from build123d import *

# Parameters (mm, degrees)
F1_DEPTH = 12.7
F4_SIZE  = 0.5
F6_R     = 7.25
F7_DEPTH = 9.3323626992
F8_SIZE  = 0.5


# Not quite as in the source:
# - a feature names something its author has since deleted; it is built from what else it names


with BuildPart() as f1:
    # F0 (on Right) → F1 (new body, symmetric)
    with BuildSketch(Plane.YZ):
        Polygon((12.7, 76.2), (-12.7, 76.2), (-12.7, 60.325), (-3.302, 60.325), (-3.302, 69.85), (0, 69.85), (0, -76.2), (12.7, -76.2), align=None)
    extrude(amount=F1_DEPTH, both=True)

    # F2 (on Right) → F3 (revolve)
    with BuildSketch(Plane.YZ):
        Polygon((-77.6932350437, -23.067179641), (-79.3034106209, -26.5202123096), (6.35, -66.4610536293), (7.9601755772, -63.0080209607), align=None)
    revolve(axis=Axis((0, -36.4767053105, -46.4906329695), (0, 0.906307787, -0.4226182617)))

    # F4
    f4_edges = [f1.edges().sort_by_distance(p)[0] for p in [
        (-12.7, 0, 76.2),
        (-12.7, 0, -3.175),
        (-12.7, 6.35, -76.2),
        (-12.7, -1.651, 69.85),
        (-12.7, -3.302, 65.0875),
        (-12.7, -12.7, 68.2625),
        (-12.7, -8.001, 60.325),
        (12.7, 6.35, -76.2),
        (12.7, 0, 76.2),
        (12.7, -12.7, 68.2625),
        (12.7, -1.651, 69.85),
        (12.7, -3.302, 65.0875),
        (12.7, -8.001, 60.325),
        (12.7, 0, -3.175),
        (0, 0, -76.2),
        (0, -12.7, 76.2),
        (0, -12.7, 60.325),
        (0, -3.302, 60.325),
    ]]
    chamfer(f4_edges, length=F4_SIZE)

    # F6 (on offset) → F7 (join, up to face)
    with BuildSketch(Plane(origin=(0, 19.834208268, -9.2488432088), x_dir=(1, 0, 0), z_dir=(0, -0.906307787, 0.4226182617))):
        with Locations((0, -57.5505444768)):
            Circle(F6_R)
    extrude(amount=-F7_DEPTH)

    # F8
    f8_edges = [f1.edges().sort_by_distance(p)[0] for p in [
        (-7.25, -4.487703, -61.40735),
    ]]
    chamfer(f8_edges, length=F8_SIZE)


solid = f1.part
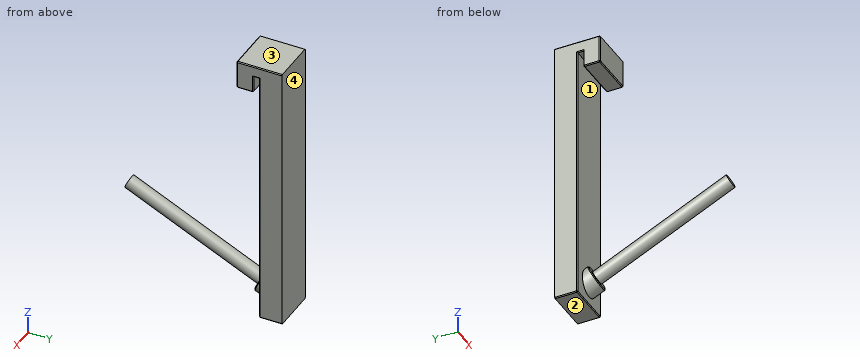
Can you work these out from the model? Positions are in its coordinate system, mm. Face numbers are marked on the shaded views. Coordinates: 2 decimals unless noted, no trailing zeros. Order: outer loops, then holes, each group sorted by start corner. A loop starts at its lowest first (then second) coordinate and runs counter-clockwise, first axis right, second up. Notation, with made-up numbers: (-16.5, 31) -> (-6.5, 31) arc R7 cw to (-6.5, 40) -> close; hole circle Ø5 at (74.25, 71.5). An arc over 180 degrees is marked (long way). Use one line per item in the form item = value.
Q1. Will these pins go through, and if not, where does the flat tip stop? P1, Ø9, axis at x = -5.5, y = -6.5, coming from the -Z side; P2, Ø2, axis at x = -5, z = -0.5, coming from the -Y side; P3, Ø1, axis at x = 2.5, y = -56, coming from the -Z side.
From the geometry:
P1 = -69.54
P2 = 0
P3 = -41.04
Q2. I need wall thicknesses on L1, parallel to Y at x = -8, z = 64; L2, parallel to Y at x = -9.5, z = 31.5; L3, parallel to Z at x = -1, y = -1.5. Which ranges of each line are inside material? Lowest first, please.
From the geometry:
L1 = -12.7 to -3.3, 0 to 12.7
L2 = 0 to 12.7
L3 = -70.72 to -55.3, 69.85 to 76.2
Q3. We'd pull the mould along Z, two halves only. Please class the marked faces 1, 2, 3 and 4: released by +Z, released by -Z, zero draft, split by the parting line, or undercut.
From the geometry:
face_1 = undercut
face_2 = released by -Z
face_3 = released by +Z
face_4 = zero draft
Q4. Imagine slicing it at A-A, the plane x = 9. List the corners of the cut face in (y, z) for me (3 decimals).
From the geometry:
outline = (-12.7, 60.825) -> (-12.2, 60.325) -> (-3.802, 60.325) -> (-3.302, 60.825) -> (-3.302, 69.85) -> (0, 69.85) -> (0, -75.7) -> (0.5, -76.2) -> (12.7, -76.2) -> (12.7, 76.2) -> (-12.2, 76.2) -> (-12.7, 75.7) -> close
Q5. Imagine slicing it at B-B, the plane z = -3. List the corners of the cut face in (x, y) for me.
From the geometry:
outline = (-12.7, 0.5) -> (-12.2, 0) -> (12.2, 0) -> (12.7, 0.5) -> (12.7, 12.7) -> (-12.7, 12.7) -> close
